Source: three-view drawing plus pictorial views. Frame: mm from the lowest corner of the part. A direction names the side the tool comes from. Give positions to 0.01 mm unless a question says otherwise; leave off trailing zeros. Loops run counter-clockwise (first coordinate to the right, second up) from the corner with the lowest first, then second, coordinate; pieces in that order, holes last. Notation, with made-up numbers: (24.25, -5) - (46.25, -5) arc R12 cw to (46.25, 17) - close; hole circle Ø10 at (-25, 41.5). An arc over 180 degrees is marked (long way). Answer as a JSON object with one key per item and string values. Group by question number.
(1) Section query D-D (x = 11). Return loops of the section in (y, z).
(2) Section query B-B (z = 21.5). Return loops of the section in (x, y), plus the area to 3 significant figures.
(3) Material intervals for L1, parallel to Y at x = 58, z = 30; L2, parallel to Z at x = 63, y = 22.5; L3, parallel to Y at x = 57.5, z = 23, sorted ascending.
(4) Section query A-A (x = 45). Count the separate pieces of the cut face and the enclosed holes in it, plus the area to 3 significant figures.
(5) Pin query (flat end, axial travel): P1, Ø20, axis at x = 45, y = 25, coming from the +Z side; P2, Ø14.5, axis at x = 80, y = 25, coming from the -Z side; P3, Ø9, axis at x = 10, z = 44, coming from the +Y side; P4, Ø3, axis at x = 17.5, z = 12.5, coming from the +Y side. Return the tip coordinate at first contact, or that it passes through.
(6) Mould query, pull axis X, two halves, no side actions, for the marked faces 1, 2 and 3. Classes: +X half, -X half, draft (parallel to the pull), parting line (faces both ways), or undercut.
(7) Access query for the marked faces 4, 5, 6, 7 and 8. Directions: +Z, -Z, +X, -X, +Y, -Y. A direction counts if a zero-diameter tool reaches every point of the face in a straight line with its end or side. Return the directions, or none.
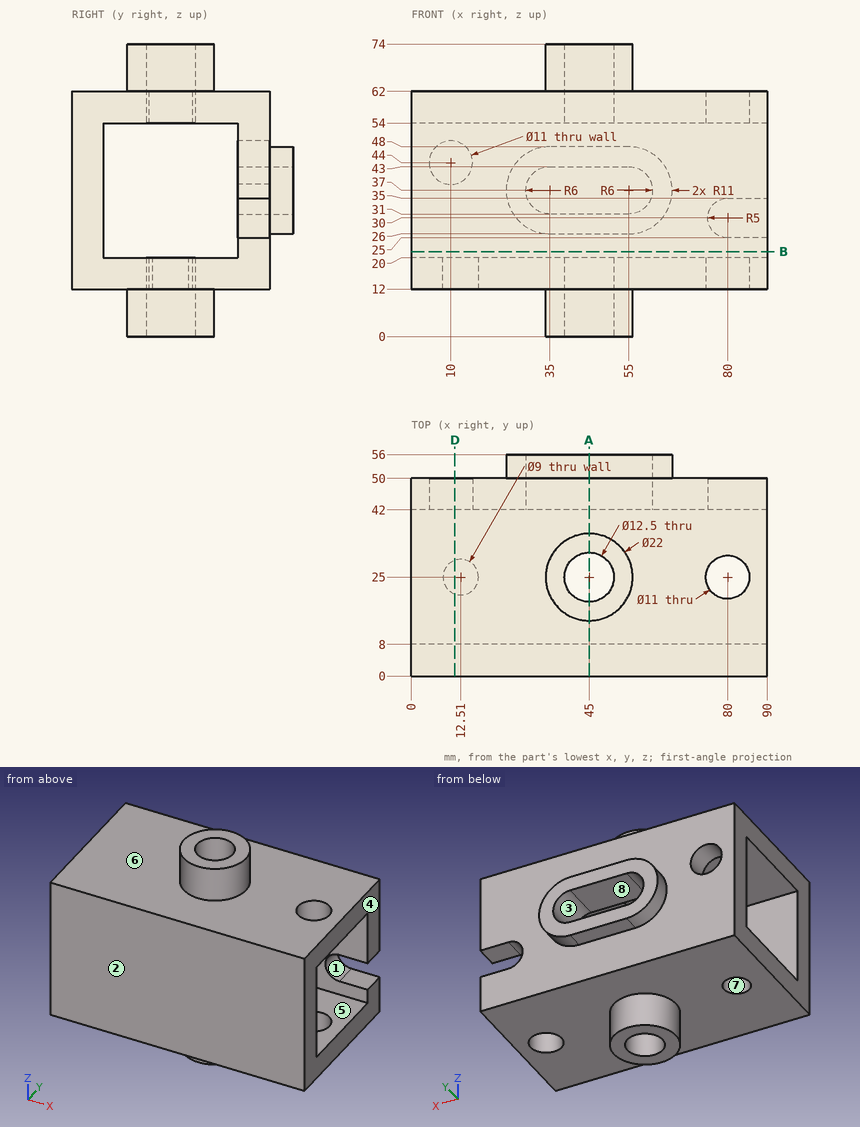
Recorded:
{
 "1": {"outline": "(0, 12) - (20.76, 12) - (20.76, 20) - (8, 20) - (8, 54) - (42, 54) - (42, 49.41) - (50, 49.41) - (50, 62) - (0, 62) - close; (29.24, 12) - (50, 12) - (50, 38.59) - (42, 38.59) - (42, 20) - (29.24, 20) - close"},
 "2": {"outline": "(0, 0) - (90, 0) - (90, 8) - (0, 8) - close; (0, 42) - (90, 42) - (90, 50) - (0, 50) - close", "area": "1,440 mm^2"},
 "3": {"L1": "y = 0 to 8, 42 to 56", "L2": "z = 12 to 20, 54 to 62", "L3": "y = 0 to 8, 42 to 50"},
 "4": {"separate pieces": "3", "enclosed holes": "0", "area": "1,340 mm^2"},
 "5": {"P1": "stops at z = 74", "P2": "stops at z = 12", "P3": "stops at y = 8", "P4": "stops at y = 50"},
 "6": {"face 1": "+X half", "face 2": "draft", "face 3": "undercut"},
 "7": {"face 4": "+Z, -Z, +X, +Y, -Y", "face 5": "+X, -X", "face 6": "+Z", "face 7": "-Z", "face 8": "+Y"}
}
